The model under review builds one solid part; all positions refer to its coordinate system, in mm. A direction names the side the tool comes from. Give positions to 0.01 mm unless a question says otherwise; leave off trailing zeros. Loops run counter-clockwise (first coordinate to the right, second up) from the corner with the lowest first, then second, coordinate; pieces in that order, holes last. Notation, with made-up numbers: (40.25, -21.5) - (65.25, -21.5) arc R8 ccw to (65.25, -15.5) - close; hole circle Ø4 at (87, 6). An arc over 180 degrees is marked (long way). Return JSON: item names as keys, results as strings. Group by question number.
from build123d import *

# Parameters (mm, degrees)
BOSS_EXTRUDE1_DEPTH = 19.05
SKETCH2_W           = 57.15
SKETCH2_H           = 25.4
BOSS_EXTRUDE2_DEPTH = 31.75
SKETCH6_W           = 38.1
SKETCH6_H           = 12.7
BOSS_EXTRUDE3_DEPTH = 25.4
CUT_EXTRUDE1_START  = -18
CUT_EXTRUDE1_DEPTH  = 33.875


with BuildPart() as part:
    # Sketch1 → Boss-Extrude1 (new body)
    with BuildSketch(Plane(origin=(0, 0, 0), x_dir=(0, 0, -1), z_dir=(1, 0, 0))):
        Polygon((-15.875, 40.443322581), (15.875, 40.443322581), (15.875, 49.968322581), (28.575, 49.968322581), (28.575, 0), (-28.575, 0), (-28.575, 49.968322581), (-15.875, 49.968322581), align=None)
    extrude(amount=BOSS_EXTRUDE1_DEPTH)

    # Sketch2 → Boss-Extrude2 (add)
    with BuildSketch(Plane(origin=(19.05, 0, 0), x_dir=(0, 0, -1), z_dir=(1, 0, 0))):
        with Locations((0, 12.7)):
            Rectangle(SKETCH2_W, SKETCH2_H)
    extrude(amount=BOSS_EXTRUDE2_DEPTH)

    # Sketch6 → Boss-Extrude3 (add)
    with BuildSketch(Plane(origin=(50.8, 0, 0), x_dir=(0, 0, -1), z_dir=(1, 0, 0))):
        with Locations((-9.525, 6.35)):
            Rectangle(SKETCH6_W, SKETCH6_H)
    extrude(amount=BOSS_EXTRUDE3_DEPTH)

    # Cut-Extrude1: read off the stored shape, not the designer's step
    # Cut-Extrude1 outline → Cut-Extrude1 (cut)
    with BuildSketch(Plane(origin=(0, 0, 0), x_dir=(1, 0, 0), z_dir=(0, 0.7999999999999996, -0.6000000000000005)).offset(CUT_EXTRUDE1_START)):
        Polygon((24, -38.94), (24, -40), (76.2, -40), (76.2, -7.62), align=None)
    extrude(amount=CUT_EXTRUDE1_DEPTH, mode=Mode.SUBTRACT)


solid = part.part
Item 1: Mouldability with a two-part tool opening along Z and no side actions: class faces 1 (the face through (9, 40.443, 0)), 2 (the face through (9, 45, 15.875)), 3 (the face through (63, 6, -9.525)), 4 (the face through (19.05, 35, 0)) as +Z half, -Z half, draft (parallel to the pull), parting line (faces both ways), or undercut.
Item 2: Take a section at C-C (z = 6). State the section outline as (x, y) points.
Item 3: For L1, parallel to X at y = 30.5, z = -14.5; L2, parallel to Y at x = 5, z = 3.5; L3, parallel to Y at x = 36, z = 19, list the stretches that pass through material, from the lowest coordinate up. Write a range as from..to.
Item 4: Take a section at D-D (y = 17). State the section outline as (x, z) points (3 decimals), then the cut area to 3 significant figures.
Item 5: For P1, Ø10, axis at y = 11.5, z = 14, coming from the +X side; P2, Ø4, axis at x = 49.5, z = 22.5, coming from the +Y side; P3, Ø2, axis at y = 27.5, z = 10, coming from the +X side; P4, Ø10, axis at x = 43.5, y = 31, coming from the +Z side, all flat-tipped, find the tip position at first contact; note any pin that passes through.
Item 6: Take a section at B-B (x = 5.5). State the section outline as (y, z) points (3 decimals).
Item 7: Take a section at A-A (y = 42.5). State the section outline as (x, z) points (3 decimals), then the cut area to 3 significant figures.
Item 8: Tool access review of faces 5 (the face through (60, 12.7, 2)), 6 (the face through (9, 45, -15.875)), 7 (the face through (51.16, 12.39, 19.01)): name each direction out of +Z, -Z, +X, -X, +Y, -Y from which nothing blocks a thin tool from reaching the whole face with its end or side.
Check sheet entries:
{
 "1": {"face 1": "undercut", "face 2": "undercut", "face 3": "-Z half", "face 4": "draft"},
 "2": {"outline": "(0, 0) - (76.2, 0) - (76.2, 4.7) - (68.2, 12.7) - (50.8, 12.7) - (50.8, 25.4) - (19.05, 25.4) - (19.05, 40.44) - (0, 40.44) - close"},
 "3": {"L1": "x = 0..19.05", "L2": "y = 0..40.44", "L3": "y = 0..25.4"},
 "4": {"outline": "(0, -28.575) - (50.8, -28.575) - (50.8, 15.825) - (33.8, 28.575) - (0, 28.575) - close", "area": "2,790 mm^2"},
 "5": {"P1": "stops at x = 67.07", "P2": "stops at y = 12.73", "P3": "stops at x = 19.05", "P4": "passes through"},
 "6": {"outline": "(0, -28.575) - (49.968, -28.575) - (49.968, -15.875) - (40.443, -15.875) - (40.443, 15.875) - (49.968, 15.875) - (49.968, 28.575) - (0, 28.575) - close"},
 "7": {"outline": "(0, -28.575) - (19.05, -28.575) - (19.05, -15.875) - (0, -15.875) - close; (0, 15.875) - (19.05, 15.875) - (19.05, 28.575) - (0, 28.575) - close", "area": "484 mm^2"},
 "8": {"face 5": "+Z, -Z, +X, +Y", "face 6": "+X, -X, +Y", "face 7": "+Z, +X, +Y"}
}
